Input: part model. Units: mm. Frame: model coordinates. A direction names the side the tool comes from. Give positions to 0.01 mm unless a question says otherwise; leave off trailing zeros. Write each loop counter-clockwise with the first axis right and the second up, starting at its lowest first coordinate (ties: lowest second). Pieces come first, ordered by that corner, then holes. Notation, with made-up numbers: (39, 16) - (93, 16) arc R28 cw to (93, 34) - close; hole circle Ø6 at (4, -5.5). An arc over 180 degrees is marked (long way). Answer as CSV lines item,"result".
Autodesk Inventor part; units mm, degrees
ref_plane "Work Plane1" through (0, 1.5, 0) normal (0, 1, 0) x (1, 0, 0)
ref_plane "YZ Plane" through (0, 0, 0) normal (1, 0, 0) x (0, 1, 0)
ref_plane "XZ Plane" through (0, 0, 0) normal (0, 1, 0) x (-1, 0, 0)
sketch "Sketch1" plane through (0, 0, 0) normal (0, 1, 0) x (-1, 0, 0)
  line L0 (15.92, 5) -> (-15.92, 5)
  line L1 (-15.92, 5) -> (-15.92, -5)
  line L2 (-15.92, -5) -> (15.92, -5)
  line L3 (15.92, -5) -> (15.92, 5)
  line L4 (15.92, 5) -> (-15.92, -5) construction
  line L5 (-15.92, 5) -> (15.92, -5) construction
  line L6 (-10.87, -4.5) -> (-12.72, -4.5)
  line L7 (-12.72, -4.5) -> (-12.72, -3.5)
  line L8 (-12.72, -3.5) -> (-10.87, -3.5)
  line L9 (-10.87, -3.5) -> (-10.87, -4.5)
  circle A0 centre (-8.42, -3.75) radius 1
  line L10 (15.92, 0) -> (-15.92, 0) construction
  line L11 (0, -5) -> (0, 5) construction
  circle A1 centre (-8.42, 3.75) radius 1
  line L12 (-10.22, -2.5) -> (-15.22, -2.5)
  line L13 (-15.22, -2.5) -> (-15.22, 2.5)
  line L14 (-15.22, 2.5) -> (-10.22, 2.5)
  line L15 (-10.22, 2.5) -> (-10.22, -2.5)
  line L16 (-1.52, -2.5) -> (-6.52, -2.5)
  line L17 (-6.52, -2.5) -> (-6.52, 2.5)
  line L18 (-6.52, 2.5) -> (-1.52, 2.5)
  line L19 (-1.52, 2.5) -> (-1.52, -2.5)
  line L20 (7.18, -2.5) -> (2.18, -2.5)
  line L21 (2.18, -2.5) -> (2.18, 2.5)
  line L22 (2.18, 2.5) -> (7.18, 2.5)
  line L23 (7.18, 2.5) -> (7.18, -2.5)
  line L24 (15.22, -2.5) -> (10.22, -2.5)
  line L25 (10.22, -2.5) -> (10.22, 2.5)
  line L26 (10.22, 2.5) -> (15.22, 2.5)
  line L27 (15.22, 2.5) -> (15.22, -2.5)
  circle A2 centre (8.42, -3.75) radius 1
  circle A3 centre (8.42, 3.75) radius 1
  line L28 (-2.57, -4.5) -> (-4.42, -4.5)
  line L29 (-4.42, -4.5) -> (-4.42, -3.5)
  line L30 (-4.42, -3.5) -> (-2.57, -3.5)
  line L31 (-2.57, -3.5) -> (-2.57, -4.5)
  line L32 (5.73, -4.5) -> (3.88, -4.5)
  line L33 (3.88, -4.5) -> (3.88, -3.5)
  line L34 (3.88, -3.5) -> (5.73, -3.5)
  line L35 (5.73, -3.5) -> (5.73, -4.5)
  line L36 (13.42, -4.5) -> (11.57, -4.5)
  line L37 (11.57, -4.5) -> (11.57, -3.5)
  line L38 (11.57, -3.5) -> (13.42, -3.5)
  line L39 (13.42, -3.5) -> (13.42, -4.5)
  point P0 (0, 0)
  dimension "d0" = 31.84
  dimension "d1" = 10
  dimension "d2" = 1.85
  dimension "d3" = 1
  dimension "d4" = 7.5
  dimension "d5" = 7.5
  dimension "d6" = 2
  dimension "d7" = 3.2
  dimension "d8" = 0.5
  dimension "d9" = 5
  dimension "d10" = 0.7
  dimension "d11" = 3.7
  dimension "d12" = 0.7
  dimension "d14" = 6.45
  dimension "d15" = 6.45
  dimension "d16" = 2.5
  dimension "d18" = 3.7
extrude "Extrusion1" add sketch "Sketch1" against normal blind 1.6 contours L3 L2 L1 L0 | L6 L7 L8 L9 | L12 L13 L14 L15 | L16 L17 L18 L19 | L20 L21 L22 L23 | L24 L25 L26 L27 | L28 L29 L30 L31 | L32 L33 L34 L35 | L36 L37 L38 L39
extrude "Extrusion2" add sketch "Sketch1" along normal blind 1.6 contours L12 L13 L14 L15 | L16 L17 L18 L19 | L20 L21 L22 L23 | L24 L25 L26 L27
extrude "Extrusion3" add sketch "Sketch1" along normal blind 0.9 contours L6 L7 L8 L9 | L28 L29 L30 L31 | L32 L33 L34 L35 | L36 L37 L38 L39
sketch "Sketch2" plane through (0, 1.6, 0) normal (0, 1, 0) x (1, 0, 0)
  line L0 (-10.22, 2.5) -> (-15.22, 2.5) construction
  line L1 (-15.22, 2.5) -> (-15.22, -2.5) construction
  line L2 (-15.22, -2.5) -> (-10.22, -2.5) construction
  line L3 (-10.22, -2.5) -> (-10.22, 2.5) construction
  line L4 (-7.18, 2.5) -> (-7.18, -2.5) construction
  line L5 (-7.18, -2.5) -> (-2.18, -2.5) construction
  line L6 (-2.18, -2.5) -> (-2.18, 2.5) construction
  line L7 (-2.18, 2.5) -> (-7.18, 2.5) construction
  line L8 (6.52, 2.5) -> (1.52, 2.5) construction
  line L9 (1.52, 2.5) -> (1.52, -2.5) construction
  line L10 (1.52, -2.5) -> (6.52, -2.5) construction
  line L11 (6.52, -2.5) -> (6.52, 2.5) construction
  line L12 (10.22, 2.5) -> (10.22, -2.5) construction
  line L13 (10.22, -2.5) -> (15.22, -2.5) construction
  line L14 (15.22, -2.5) -> (15.22, 2.5) construction
  line L15 (15.22, 2.5) -> (10.22, 2.5) construction
  circle A0 centre (-12.72, 0) radius 1.75
  circle A1 centre (-4.68, 0) radius 1.75
  circle A2 centre (4.02, 0) radius 1.75
  circle A3 centre (12.72, 0) radius 1.75
  line L16 (-15.22, -2.5) -> (-15.22, 2.5) construction
  line L17 (-15.22, 1.5) -> (-14.22, 2.5)
  line L18 (-15.22, 2.5) -> (-10.22, 2.5) construction
  line L19 (-15.22, 2.5) -> (-15.22, 1.5)
  line L20 (-15.22, 2.5) -> (-14.22, 2.5)
  line L21 (-7.18, 2.5) -> (-7.18, 1.5)
  line L22 (-7.18, -2.5) -> (-7.18, 2.5) construction
  line L23 (-7.18, 2.5) -> (-2.18, 2.5) construction
  line L24 (-7.18, 2.5) -> (-6.18, 2.5)
  line L25 (-7.18, 1.5) -> (-6.18, 2.5)
  line L26 (1.52, 2.5) -> (1.52, 1.5)
  line L27 (1.52, 1.5) -> (2.52, 2.5)
  line L28 (1.52, -2.5) -> (1.52, 2.5) construction
  line L29 (2.52, 2.5) -> (1.52, 2.5)
  line L30 (10.22, 2.5) -> (10.22, 1.5)
  line L31 (10.22, -2.5) -> (10.22, 2.5) construction
  line L32 (10.22, 2.5) -> (15.22, 2.5) construction
  line L33 (10.22, 2.5) -> (11.22, 2.5)
  line L34 (10.22, 1.5) -> (11.22, 2.5)
  point P0 (0, 0)
  dimension "d25" = 3.5
  dimension "d26" = 45
  dimension "d27" = 1
extrude "Extrusion4" cut sketch "Sketch2" against normal blind 0.2 contours L19 L20 L17 | L24 L25 L21 | L29 L27 L26 | L33 L34 L30
extrude "Extrusion5" cut sketch "Sketch2" against normal blind 0.8 contours A0 | A1 | A2 | A3
ref_plane "Work Plane1" through (0, 1.5, 0) normal (0, 1, 0) x (1, 0, 0)
sketch "Sketch3" plane through (0, 1.5, 0) normal (0, 1, 0) x (1, 0, 0)
  circle A0 centre (-12.72, 0) radius 1.75
  circle A1 centre (-4.68, 0) radius 1.75
  circle A2 centre (4.02, 0) radius 1.75
  circle A3 centre (12.72, 0) radius 1.75
  point P0 (0, 0)
extrude "Extrusion7" add sketch "Sketch3" against normal up to next
equation "\"d12\" = d10"
equation "\"d15\" = d14"
equation "\"d18\" = d11"
properties part number "LED WS2812B"
Item 1: Ray query, line 1 (Z direction, x = -8.42, y = -0.25); line 2 (X direction, y = 0.9, z = 1.25); line 3 (X direction, y = -0.4, z = 3.25). Return the intervals inside material, ascending. Write a range as from..to.
The answers:
line 1,"-5..-4.75, -2.75..2.75, 4.75..5"
line 2,"-15.22..-10.22, -7.18..-2.18, 1.52..6.52, 10.22..15.22"
line 3,"-15.92..-9.29, -7.55..7.55, 9.29..15.92"
Item 2: Contact query for flat-ended pins moving along their axis: pin 1 (3 mm diameter, centred on x = 12.72, z = 0, fed in from +Y); pin 2 (1.1 mm diameter, centred on x = -5, z = -4, fed in from +Y); pin 3 (2 mm diameter, centred on x = -8.5, z = -3.5, fed in from +Y). Output: stop coordinate, or through.
The answers:
pin 1,"y = 1.5"
pin 2,"y = 0.9"
pin 3,"y = 0"
Item 3: Reachability of faces 1 (the face through (4, 1.5, 0)), 2 (the face through (4, 0.9, -4)), 3 (the face through (-5, 1, -2.5)), 4 (the face through (-5.73, 0.4, -4)) from +Z, -Z, +X, -X, +Y, -Y: full face, straight path, thin tool, end or side. Return the list, or none.
The answers:
face 1,"+Y"
face 2,"-Z, +X, -X, +Y"
face 3,"+X, -X, +Y"
face 4,"-Z, +Y"
Item 4: Cut plane C-C on x = 8.42. Return the cut outline in (y, z).
The answers:
outline,"(-1.6, -5) - (0, -5) - (0, -4.75) - (-1.6, -4.75) - close; (-1.6, -2.75) - (0, -2.75) - (0, 2.75) - (-1.6, 2.75) - close; (-1.6, 4.75) - (0, 4.75) - (0, 5) - (-1.6, 5) - close"
Item 5: Mould query, pull axis X, two halves, no side actions, for faces 5 (the face through (15.22, 1, 0)), 6 (the face through (3.5, 0.4, -4.5)), 7 (the face through (1.52, 1, 0)), 8 (the face through (10.87, 0.4, -4)). Classes: +X half, -X half, draft (parallel to the pull), parting line (faces both ways), or undercut.
The answers:
face 5,"+X half"
face 6,"draft"
face 7,"undercut"
face 8,"undercut"
Item 6: Cut plane D-D on x = -12.72. Return the cut outline in (y, z).
The answers:
outline,"(-1.6, -5) - (0, -5) - (0, -4.5) - (0.9, -4.5) - (0.9, -3.5) - (0, -3.5) - (0, -2.5) - (1.6, -2.5) - (1.6, -1.75) - (1.5, -1.75) - (1.5, 1.75) - (1.6, 1.75) - (1.6, 2.5) - (0, 2.5) - (0, 5) - (-1.6, 5) - close"
Item 7: Cut plane B-B on y = 0.3. Count the separate pieces of the cut face and the enclosed holes in it, plus the area to 3 significant figures.
The answers:
separate pieces,"8"
enclosed holes,"0"
area,"107 mm²"
Item 8: Cut plane A-A on z = 3.75. Return the cut outline in (x, y).
The answers:
outline,"(-15.92, -1.6) - (-9.42, -1.6) - (-9.42, 0) - (-15.92, 0) - close; (-7.42, -1.6) - (7.42, -1.6) - (7.42, 0) - (-7.42, 0) - close; (9.42, -1.6) - (15.92, -1.6) - (15.92, 0) - (9.42, 0) - close"
